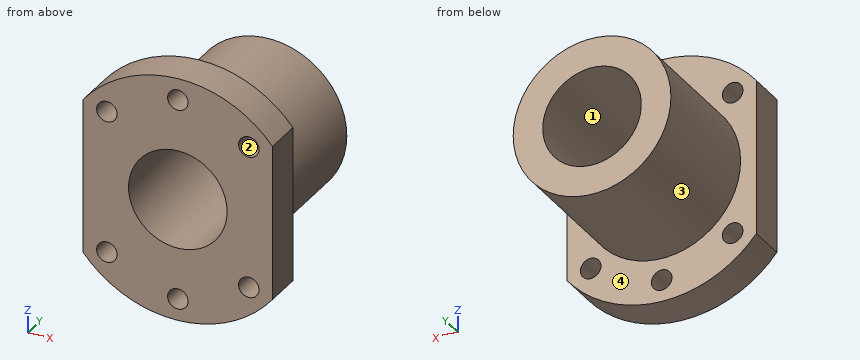
from build123d import *

# Parameters (mm, degrees)
SKETCH1_R           = 2.6
BOSS_EXTRUDE1_DEPTH = 10
SKETCH2_R           = 20
BOSS_EXTRUDE2_DEPTH = 34
CUT_EXTRUDE1_REACH  = 46
SKETCH3_R           = 12.5


with BuildPart() as part:
    # Sketch1 → Boss-Extrude1 (new body)
    with BuildSketch(Plane(origin=(0, 0, 0), x_dir=(1, 0, 0), z_dir=(0, 1, 0))):
        with BuildLine():
            Line((-24, 19.62141687), (-24, -19.62141687))
            ThreePointArc((-24, -19.62141687), (0, -31), (24, -19.62141687))
            Line((24, -19.62141687), (24, 19.62141687))
            ThreePointArc((24, 19.62141687), (0, 31), (-24, 19.62141687))
        make_face()
        with Locations((18, 18)):
            Circle(SKETCH1_R, mode=Mode.SUBTRACT)
        with Locations((0, 25.5)):
            Circle(SKETCH1_R, mode=Mode.SUBTRACT)
        with Locations((-18, 18)):
            Circle(SKETCH1_R, mode=Mode.SUBTRACT)
        with Locations((-18, -18)):
            Circle(SKETCH1_R, mode=Mode.SUBTRACT)
        with Locations((18, -18)):
            Circle(SKETCH1_R, mode=Mode.SUBTRACT)
        with Locations((0, -25.5)):
            Circle(SKETCH1_R, mode=Mode.SUBTRACT)
    extrude(amount=BOSS_EXTRUDE1_DEPTH)

    # Sketch2 → Boss-Extrude2 (add)
    with BuildSketch(Plane(origin=(0, 10, 0), x_dir=(1, 0, 0), z_dir=(0, 1, 0))):
        Circle(SKETCH2_R)
    extrude(amount=BOSS_EXTRUDE2_DEPTH)

    # Sketch3 → Cut-Extrude1 (cut, up to next)
    with BuildSketch(Plane(origin=(0, 44, 0), x_dir=(1, 0, 0), z_dir=(0, 1, 0)), mode=Mode.PRIVATE) as cut_extrude1_sk1:
        Circle(SKETCH3_R)
    cut_extrude1_tool1 = extrude(cut_extrude1_sk1.sketch, amount=-CUT_EXTRUDE1_REACH, mode=Mode.PRIVATE) & part.part
    add(cut_extrude1_tool1.solids().sort_by_distance((0, 44, 0))[0], mode=Mode.SUBTRACT)


solid = part.part
The listing builds one solid part. Answer for the finished solid, in the listing's coordinates (mm). Face numbers are marked on the shaded views. Round coordinates to 2 decimals unless told otherwise and drop trailing zeros. Order: outer loops, then holes, each group sorted by start corner. A loop starts at its lowest first (then second) coordinate and runs counter-clockwise, first axis right, second up. Notation, with made-up numbers: (52.5, 39) - (92.5, 39) arc R20 ccw to (92.5, 61) - close; hole circle Ø7 at (-27.5, -10.5). An arc over 180 degrees is marked (long way). Write item = value, one per line. Start each with the question number.
1) Section B-B, the plane z = 10.5 is taken. Write down the section's boundary in (x, y).
2) Straight lines are drawn through the part: L1, parallel to X at y = 3.5, z = 18; L2, parallel to Z at x = 18, y = 4; L3, parallel to X at y = 22, z = 0. For each, find the intervals that lie inside material, in ascending order.
3) Section C-C, the plane z = 18 is taken. Write down the section's boundary in (x, y), plus the area to 3 significant figures.
4) Given pin 1 (4 mm diameter, centred on y = 27, z = 1, fed in from +X); pin 2 (8.5 mm diameter, centred on x = 18, z = -18, fed in from +Y); pin 3 (10 mm diameter, centred on y = 36.5, z = -18.5, fed in from -X); pin 4 (8 mm diameter, centred on x = -9, z = -4.5, fed in from -Y), each flat-ended and moving along its own axis, determine where each tip first touches the part or whether it passes through.
5) Section D-D, the plane y = 37.5 is taken. Write down the section's boundary in (x, z).
6) Section A-A, the plane x = 0 is taken. Write down the section's boundary in (y, z).
7) For a pull along Z with two mould halves and no side action, classify the marked faces 1, 2, 3 and 4 as released by +Z, released by -Z, zero draft, split by the parting line, or undercut.
Results list:
q1.outline = (-24, 0) - (-6.78, 0) - (-6.78, 44) - (-17.02, 44) - (-17.02, 10) - (-24, 10) - close; (6.78, 0) - (24, 0) - (24, 10) - (17.02, 10) - (17.02, 44) - (6.78, 44) - close
q2.L1 = -24 to -20.6, -15.4 to 15.4, 20.6 to 24
q2.L2 = -25.24 to -20.6, -15.4 to 15.4, 20.6 to 25.24
q2.L3 = -20 to -12.5, 12.5 to 20
q3.outline = (-24, 0) - (-20.6, 0) - (-20.6, 10) - (-24, 10) - close; (-15.4, 0) - (15.4, 0) - (15.4, 10) - (8.72, 10) - (8.72, 44) - (-8.72, 44) - (-8.72, 10) - (-15.4, 10) - close; (20.6, 0) - (24, 0) - (24, 10) - (20.6, 10) - close
q3.area = 969 mm^2
q4.pin_1 = 20
q4.pin_2 = 10
q4.pin_3 = -14.76
q4.pin_4 = 0
q5.outline = circle Ø40 at (0, 0); hole circle Ø25 at (0, 0)
q6.outline = (0, -31) - (10, -31) - (10, -28.1) - (0, -28.1) - close; (0, -22.9) - (10, -22.9) - (10, -20) - (44, -20) - (44, -12.5) - (0, -12.5) - close; (0, 12.5) - (44, 12.5) - (44, 20) - (10, 20) - (10, 22.9) - (0, 22.9) - close; (0, 28.1) - (10, 28.1) - (10, 31) - (0, 31) - close
q7.face_1 = undercut
q7.face_2 = undercut
q7.face_3 = split by the parting line
q7.face_4 = zero draft
